The figure shows three views and two pictorial views of one solid part (mm, origin at its lowest corner). Answer the questions. Round coordinates to 2 decimals unless told otherwise and drop trailing zeros. Write each loop counter-clockwise with the first axis right and the second up, starting at its lowest first coordinate (ties: lowest second). Pieces come first, ordered by that corner, then holes.
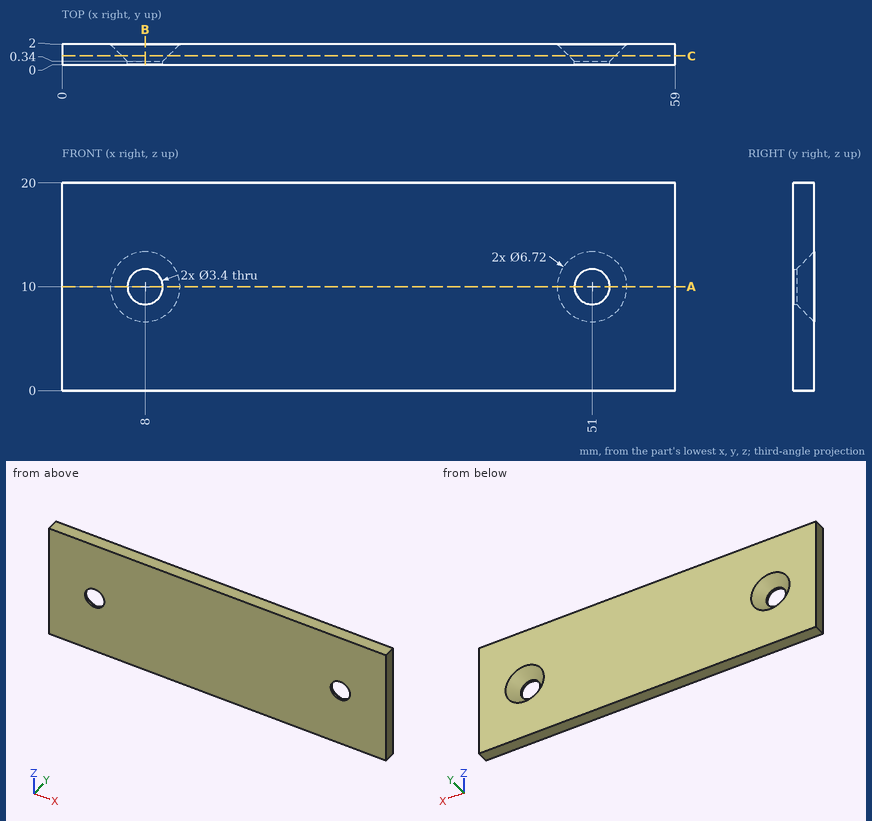
Q1. Section C-C (y = 0.85) is taken. Determine the outline of the cut face in (x, z).
Verdict:
outline: (0, 0) - (59, 0) - (59, 20) - (0, 20) - close; hole circle Ø4.42 at (8, 10); hole circle Ø4.42 at (51, 10)
Q2. Section A-A (z = 10) is taken. Determine the outline of the cut face in (x, y), then the cut area to 3 significant figures.
Verdict:
outline: (0, 0) - (6.3, 0) - (6.3, 0.34) - (4.64, 2) - (0, 2) - close; (9.7, 0) - (49.3, 0) - (49.3, 0.34) - (47.64, 2) - (11.36, 2) - (9.7, 0.34) - close; (52.7, 0) - (59, 0) - (59, 2) - (54.36, 2) - (52.7, 0.34) - close
area: 98.9 mm2
Q3. A flat-ended cylindrical pin translates along its axis: pin 1 Ø12 at (x, z) = (49, 13.5) entering from -Y. Find the tip coordinate at first contact, or state that the pin passes through.
Verdict:
pin 1: stops at y = 0
Q4. Section B-B (x = 8) is taken. Determine the outline of the cut face in (y, z).
Verdict:
outline: (0, 0) - (2, 0) - (2, 6.64) - (0.34, 8.3) - (0, 8.3) - close; (0, 11.7) - (0.34, 11.7) - (2, 13.36) - (2, 20) - (0, 20) - close
Q5. Straight lines are drawn through the part: probe 1 along X at (y, z) = (0.2, 10); probe 2 along Z at (x, y) = (8, 0.2); probe 3 along X at (y, z) = (0.4, 8.5). For each, find the intervals that lie inside material, in ascending order.
Verdict:
probe 1: x = 0 to 6.3, 9.7 to 49.3, 52.7 to 59
probe 2: z = 0 to 8.3, 11.7 to 20
probe 3: x = 0 to 7.08, 8.92 to 50.08, 51.92 to 59
